Read the model definition and answer for the solid it produces. Units are mm, in the model's axes. Coordinates: 2 decimals unless noted, no trailing zeros. Order: outer loops, then holes, each group sorted by start corner. A loop starts at its lowest first (then second) coordinate and runs counter-clockwise, first axis right, second up.
Autodesk Inventor part; units mm, degrees
ref_plane "YZ Plane" through (0, 0, 0) normal (1, 0, 0) x (0, 1, 0)
ref_plane "XZ Plane" through (0, 0, 0) normal (0, 1, 0) x (-1, 0, 0)
ref_plane "XY Plane" through (0, 0, 0) normal (0, 0, 1) x (1, 0, 0)
sketch "Sketch1" plane through (0, 0, 0) normal (0, 0, 1) x (1, 0, 0)
  line L0 (-139.7, -139.7) -> (139.7, -139.7)
  line L1 (139.7, -139.7) -> (139.7, 139.7)
  line L2 (139.7, 139.7) -> (-139.7, 139.7)
  line L3 (-139.7, 139.7) -> (-139.7, -139.7)
  line L4 (-139.7, -139.7) -> (139.7, 139.7) construction
  line L5 (139.7, -139.7) -> (-139.7, 139.7) construction
  point P0 (0, 0)
  dimension "d0" = 279.4
extrude "Extrusion1" add sketch "Sketch1" along normal blind 2.54
sketch "Sketch3" plane through (0, 0, 2.54) normal (0, 0, 1) x (1, 0, 0)
  line L0 (-107.95, 114.3) -> (-95.25, 114.3)
  line L1 (-95.25, 114.3) -> (-95.25, -114.3)
  line L2 (-95.25, -114.3) -> (-107.95, -114.3)
  line L3 (-107.95, -114.3) -> (-107.95, 114.3)
  line L4 (-107.95, 114.3) -> (-95.25, -114.3) construction
  line L5 (-95.25, 114.3) -> (-107.95, -114.3) construction
  line L6 (0, 0) -> (-101.6, 0)
  line L7 (-139.7, 139.7) -> (-139.7, -139.7)
  line L8 (-139.7, -139.7) -> (139.7, -139.7)
  dimension "d11" = 12.7
  dimension "d12" = 31.75
  dimension "d13" = 25.4
extrude "Extrusion2" cut sketch "Sketch3" against normal up to next
pattern_linear "Rectangular Pattern1" count 9 spacing 25.4 along (1, 0, 0) of "Extrusion2"
properties part number "screen"
1) A straight line is drawn through the part: line 1 (Y direction, x = -26.5, z = 0.6). Find the intervals that lie inside material, in ascending order.
A:
line 1: y = -139.7 to -114.3, 114.3 to 139.7
2) A flat-ended cylindrical pin translates along its axis: pin 1 Ø12 at (x, y) = (-51, 76) entering from +Z. Find the tip coordinate at first contact, or state that the pin passes through.
A:
pin 1: passes through
3) A cutting plane is placed at B-B, the plane y = 46. State how many separate pieces and enclosed holes the cut face has, and give its area (3 significant figures).
A:
separate pieces: 10
enclosed holes: 0
area: 419 mm2
4) A cutting plane is placed at A-A, the plane x = 52.5. Determine the outline of the cut face in (y, z).
A:
outline: (-139.7, 0) - (-114.3, 0) - (-114.3, 2.54) - (-139.7, 2.54) - close; (114.3, 0) - (139.7, 0) - (139.7, 2.54) - (114.3, 2.54) - close
